Part model, mm, in its own coordinate system. Face numbers are marked on the shaded views. A direction names the side the tool comes from. Give positions to 0.01 mm unless a question says otherwise; leave off trailing zeros. Loops run counter-clockwise (first coordinate to the right, second up) from the corner with the lowest first, then second, coordinate; pieces in that order, holes last. Notation, with made-up numbers: (2.5, -28.75) -> (33.5, -28.75) arc R22 ccw to (33.5, -6.75) -> close; hole circle Ø8 at (31, 17). An arc over 180 degrees is marked (long way). Write item = value, one per line.
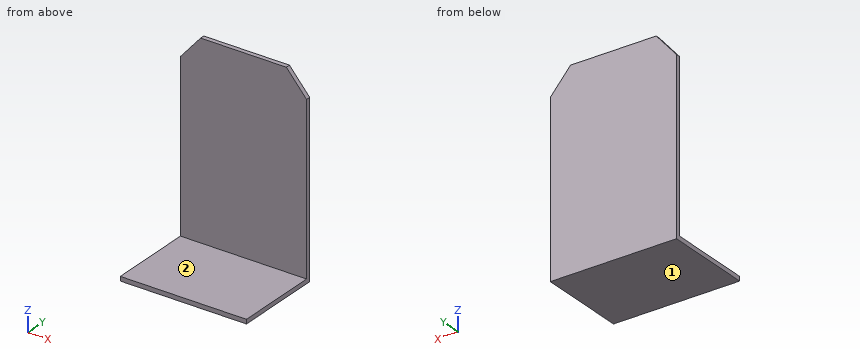
from build123d import *

# Parameters (mm, degrees)
SKETCH1_W               = 34.671
SKETCH1_H               = 52.197
BOSS_EXTRUDE1_DEPTH     = 1.1938
SKETCH3_W               = 34.671
SKETCH3_H               = 24.384
BOSS_EXTRUDE2_DEPTH     = 1.1938
CUT_EXTRUDE1_DEPTH      = 68.752794346
CUT_EXTRUDE1_DEPTH_BACK = 68.752794346


with BuildPart() as part:
    # Sketch1 → Boss-Extrude1 (new body)
    with BuildSketch(Plane(origin=(0, 0, 0), x_dir=(1, 0, 0), z_dir=(0, 1, 0))):
        with Locations((17.3355, 26.0985)):
            Rectangle(SKETCH1_W, SKETCH1_H)
    extrude(amount=BOSS_EXTRUDE1_DEPTH)

    # Sketch3 → Boss-Extrude2 (add)
    with BuildSketch(Plane(origin=(0, 0, -52.197), x_dir=(-1, 0, 0), z_dir=(0, 0, -1))):
        with Locations((-17.3355, -10.9982)):
            Rectangle(SKETCH3_W, SKETCH3_H)
    extrude(amount=BOSS_EXTRUDE2_DEPTH)

    # Sketch4 → Cut-Extrude1 (cut, two sides: drawn at the far end of the back side and taken through both)
    with BuildSketch(Plane(origin=(0, 0, 0), x_dir=(-1, 0, 0), z_dir=(0, -1, 0)).offset(-CUT_EXTRUDE1_DEPTH_BACK)):
        Polygon((0, 6.4516), (-5.5626, 0), (0, 0), align=None)
        Polygon((-29.1084, 0), (-34.671, 6.4516), (-34.671, 0), align=None)
    extrude(amount=CUT_EXTRUDE1_DEPTH + CUT_EXTRUDE1_DEPTH_BACK, mode=Mode.SUBTRACT)


solid = part.part
1) Slice it at B-B, the plane z = -45. List the corners of the cut face in (x, y).
Resolved:
outline = (0, 0) -> (34.67, 0) -> (34.67, 1.19) -> (0, 1.19) -> close
2) Slice it at C-C, the plane y = -21.5. List the corners of the cut face in (x, z), and give its area (3 significant figures).
Resolved:
outline = (0, -53.39) -> (34.67, -53.39) -> (34.67, -52.2) -> (0, -52.2) -> close
area = 41.4 mm²
3) Drop flat-ended pins along their axis: P1, Ø5, axis at x = 16.5, z = -21, coming from the -Y side; P2, Ø11.5, axis at x = 9.5, y = -14.5, coming from the +Z side. Give the stop position or say it passes through.
Resolved:
P1 = 0
P2 = -52.2
4) Drill centre lines: line 1 along Y through (x, z) = (33, -5); line 2 along Z through (x, y) = (3, -5). Where is each one in solid material? Low to high. Write a range as [from, to].
Resolved:
line_1 = [0, 1.19]
line_2 = [-53.39, -52.2]
5) Which spindle directions (+Z, -Z, +X, -X, +Y, -Y) get a long thin tool onto all of the face, cutting with end or side? Do the marked faces 1 and 2. Say none if no direction does.
Resolved:
face_1 = -Z, +X, -X, +Y, -Y
face_2 = +Z, +X, -X, -Y
6) Slice it at D-D, the plane x = 4. List the corners of the cut face in (y, z), and give its area (3 significant figures).
Resolved:
outline = (-23.19, -53.39) -> (1.19, -53.39) -> (1.19, -1.81) -> (0, -1.81) -> (0, -52.2) -> (-23.19, -52.2) -> close
area = 89.3 mm²
7) Slice it at A-A, the plane x = 8.5. List the corners of the cut face in (y, z).
Resolved:
outline = (-23.19, -53.39) -> (1.19, -53.39) -> (1.19, 0) -> (0, 0) -> (0, -52.2) -> (-23.19, -52.2) -> close
